```python
from build123d import *

# Parameters (mm, degrees)
F3_DEPTH = 250
F4_W     = 35
F4_H     = 75


# Not quite as in the source:
# - a pattern or mirror of a feature is missing from the dataset's text; its kind, count and spacing are read off the source's solid
# - the program builds the solid bodies; features that only make, move or delete a surface that nothing else refers to are left out


with BuildPart() as f3:
    # F2 (on Right) → F3 (new body, symmetric)
    with BuildSketch(Plane.YZ):
        Polygon((-500, 313.7653336856), (0, 447.7399299012), (0, 483.9745962156), (-500, 350), align=None)
    extrude(amount=F3_DEPTH, both=True)

    # F4 (on Top) → F5 (join, up to the next surface of F3)
    with BuildSketch(Plane.XY):
        with Locations((232.5, -462.5)):
            Rectangle(F4_W, F4_H)
    f5 = extrude(until=Until.NEXT)

    # F5_copies: F5 across plane
    add(f5.mirror(Plane(origin=(0, 0, 0), x_dir=(0, 0, -1), z_dir=(-1, 0, 0))))


solid = f3.part
```
Geometry: final body of the model. Coordinates: model frame, mm. A direction names the side the tool comes from. Give positions to 0.01 mm unless a question says otherwise; leave off trailing zeros. Loops run counter-clockwise (first coordinate to the right, second up) from the corner with the lowest first, then second, coordinate; pieces in that order, holes last. Notation, with made-up numbers: (24.25, 38) -> (52.25, 38) arc R30 cw to (52.25, 63) -> close; hole circle Ø6 at (77, -14). An arc over 180 degrees is marked (long way). Use CSV: the item, a comma, the result in double quotes.
(1) Cut plane D-D (y = -107.5). Output: boundary loops of the cut face in (x, z).
From the geometry:
outline,"(-250, 418.94) -> (250, 418.94) -> (250, 455.17) -> (-250, 455.17) -> close"
(2) Access query for faces 1 (the face through (232, -425, 165)), 2 (the face through (4, 0, 466)). Directions: +Z, -Z, +X, -X, +Y, -Y. A direction counts if a zero-diameter tool reaches every point of the face in a straight line with its end or side. Return the directions, or none.
From the geometry:
face 1,"-Z, +X, -X, +Y"
face 2,"+Z, -Z, +X, -X, +Y"
(3) First-contact query: P1, Ø8, axis at x = -46.5, y = -332, coming from the +Z side; P2, Ø1.5, axis at x = 77.5, y = -69.5, coming from the +Z side; P3, Ø6, axis at x = -153.5, y = -215.5, coming from the +Z side. Flat tips, straight axial feed; report the tip coordinate or a pass-through.
From the geometry:
P1,"z = 396.09"
P2,"z = 465.55"
P3,"z = 427.04"
(4) Cut plane C-C (x = -195). Output: boundary loops of the cut face in (y, z), plus the area to 3 significant figures.
From the geometry:
outline,"(-500, 313.77) -> (0, 447.74) -> (0, 483.97) -> (-500, 350) -> close"
area,"18,100 mm^2"
(5) Cut plane B-B (z = 326.5). Output: boundary loops of the cut face in (x, y), plus the area to 3 significant figures.
From the geometry:
outline,"(-250, -500) -> (250, -500) -> (250, -425) -> (215, -425) -> (215, -452.47) -> (-215, -452.47) -> (-215, -425) -> (-250, -425) -> close"
area,"25,700 mm^2"
(6) Cut plane A-A (z = 82.5). Output: boundary loops of the cut face in (x, y).
From the geometry:
outline,"(-250, -500) -> (-215, -500) -> (-215, -425) -> (-250, -425) -> close; (215, -500) -> (250, -500) -> (250, -425) -> (215, -425) -> close"
(7) Ray query, line 1 along X through (y, z) = (-475, 291); line 2 along Y through (x, z) = (-222, 126); line 3 along Z through (x, y) = (154, -470). Return the intervals inside material, ascending. Write a range as [from, to].
From the geometry:
line 1,"[-250, -215], [215, 250]"
line 2,"[-500, -425]"
line 3,"[321.8, 358.04]"
(8) Pull-direction query (X, two-part tool) for faces 3 (the face through (-17, -500, 317)), 4 (the face through (-250, -436, 259)), 5 (the face through (215, -463, 165)); classes: released by +X, released by -X, zero draft, split by the parting line, or undercut.
From the geometry:
face 3,"zero draft"
face 4,"released by -X"
face 5,"undercut"
